For this review, use the dimensioned drawing (mm, ordinates from the lowest corner) and the shaded views. A direction names the side the tool comes from. Give positions to 0.01 mm unless a question says otherwise; leave off trailing zeros. Write each loop counter-clockwise with the first axis right and the second up, starting at its lowest first coordinate (ties: lowest second). Pieces come first, ordered by that corner, then holes. Notation, with made-up numbers: M 82.25,11 L 100.25,11 A20 ccw 100.25,28 Z; hole C 49,89.25 d9. An arc over 180 degrees is marked long. Use a Markdown table: item, result. Add a question column.
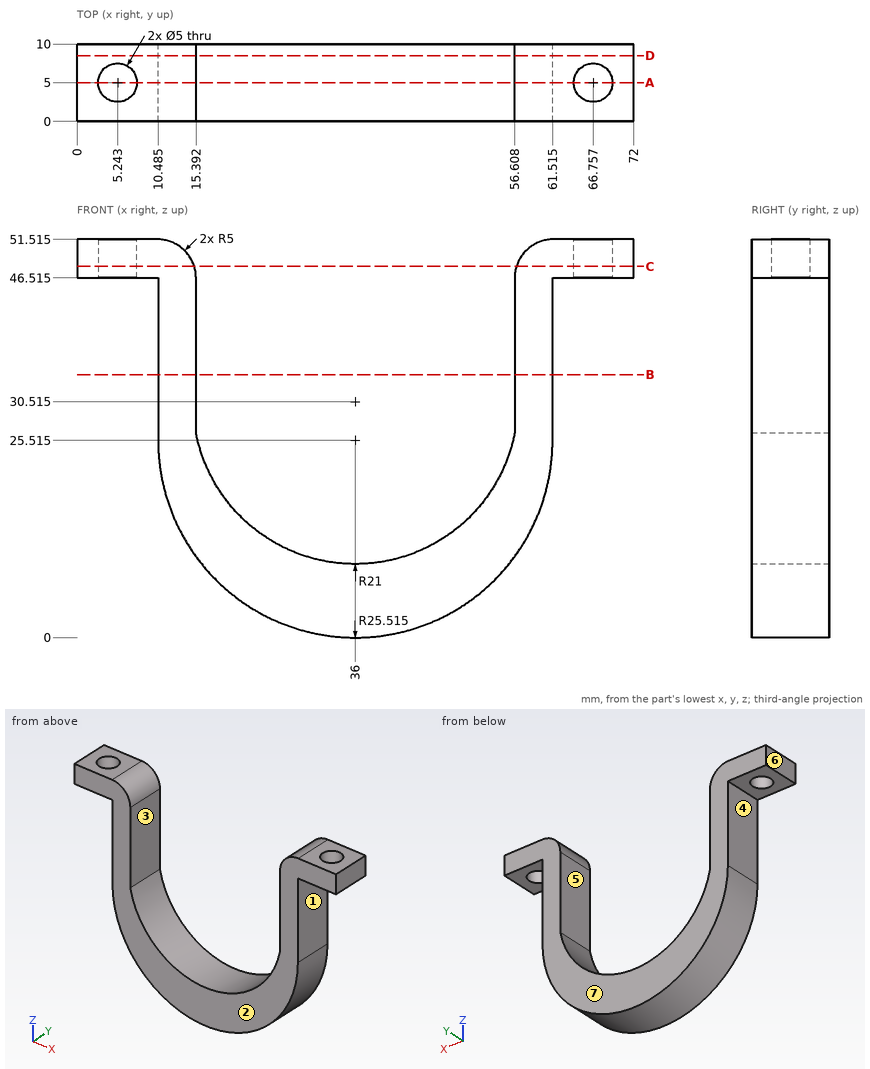
(1) Add section B-B on z = 34. Give the boundary of the cut face in (x, y) (1 decimal).
(2) Add section A-A on y = 5. Give the boundary of the cut face in (x, z) (1 decimal).
(3) The part is to be moulded in two halves that separate along X. For the marked faces 5, 6 and 7, say which applies: released by +X, released by -X, zero draft, split by the parting line, or undercut.
(4) Machinability: for the marked faces 1, 2, 3 and 4, which of the approach directions +Z, -Z, +X, -X, +Y, -Y give a long, thin tool a straight path to every point of the face, cutting with its end or side? Answer none if there is none.
(5) For pin 1 (3 mm diameter, centred on x = 5, y = 6.5, fed in from -Z) (1 decimal); pin 2 (1.5 mm diameter, centred on y = 8.5, z = 16.5, fed in from +X); pin 3 (3 mm diameter, centred on x = 66.76, y = 5, fed in from +Z); pin 4 (2 mm diameter, centred on y = 9, z = 19, fed in from +X), all flat-tipped, find the tip position at first contact; note any pin that passes through.
(6) Add section C-C on z = 48. Give the boundary of the cut face in (x, y).
(7) Wall thickness on L1, parallel to X at y = 2.25, z = 42 (1 decimal); L2, parallel to X at y = 2.75, z = 15; L3, parallel to Z at x = 65.5, y = 0.5 (1 decimal): over which ranges is each line inside the solid? List them lowest first.
(8) Add section D-D on y = 8.5. Give the boundary of the cut face in (x, z) (1 decimal).
From the geometry:
| question | item | result |
|---|---|---|
| 1 | outline | M 10.5,0 L 15.4,0 L 15.4,10 L 10.5,10 Z; M 56.6,0 L 61.5,0 L 61.5,10 L 56.6,10 Z |
| 2 | outline | M 0,46.5 L 2.7,46.5 L 2.7,51.5 L 0,51.5 Z; M 7.7,46.5 L 10.5,46.5 L 10.5,25.5 A25.5 ccw 61.5,25.5 L 61.5,46.5 L 64.3,46.5 L 64.3,51.5 L 61.6,51.5 A5 ccw 56.6,46.5 L 56.6,26.5 A21 cw 15.4,26.5 L 15.4,46.5 A5 ccw 10.4,51.5 L 7.7,51.5 Z; M 69.3,46.5 L 72,46.5 L 72,51.5 L 69.3,51.5 Z |
| 3 | face 5 | undercut |
| 3 | face 6 | released by -X |
| 3 | face 7 | zero draft |
| 4 | face 1 | -Z, +X, +Y, -Y |
| 4 | face 2 | +Z, -Z, +X, -X, -Y |
| 4 | face 3 | +Z, +Y, -Y |
| 4 | face 4 | -Z, -X, +Y, -Y |
| 5 | pin 1 | stops at z = 46.5 |
| 5 | pin 2 | stops at x = 60.14 |
| 5 | pin 3 | passes through |
| 5 | pin 4 | stops at x = 60.91 |
| 6 | outline | M 0,0 L 15.17,0 L 15.17,10 L 0,10 Z; M 56.83,0 L 72,0 L 72,10 L 56.83,10 Z; hole C 5.24,5 d5; hole C 66.76,5 d5 |
| 7 | L1 | x = 10.5 to 15.4, 56.6 to 61.5 |
| 7 | L2 | x = 12.75 to 21.85, 50.15 to 59.25 |
| 7 | L3 | z = 46.5 to 51.5 |
| 8 | outline | M 0,46.5 L 10.5,46.5 L 10.5,25.5 A25.5 ccw 61.5,25.5 L 61.5,46.5 L 72,46.5 L 72,51.5 L 61.6,51.5 A5 ccw 56.6,46.5 L 56.6,26.5 A21 cw 15.4,26.5 L 15.4,46.5 A5 ccw 10.4,51.5 L 0,51.5 Z |
